```python
from build123d import *

# Parameters (mm, degrees)
F1_DEPTH = 2
F3_DEPTH = 26
F4_R     = 5


with BuildPart() as f1:
    # F0 (on Front) → F1 (new body)
    with BuildSketch(Plane.XZ):
        with BuildLine():
            Line((-15.958655, 29.411045), (-23, 0))
            Line((-23, 0), (23, 0))
            Line((23, 0), (15.958655, 29.411045))
            ThreePointArc((15.958655, 29.411045), (0, 42), (-15.958655, 29.411045))
        make_face()
        with BuildLine():
            Line((-9.25, 20.25), (-9.25, 26.75))
            ThreePointArc((-9.25, 26.75), (0, 36), (9.25, 26.75))
            Line((9.25, 26.75), (9.25, 20.25))
            ThreePointArc((9.25, 20.25), (0, 11), (-9.25, 20.25))
        make_face(mode=Mode.SUBTRACT)
    extrude(amount=F1_DEPTH)

    # F2 (on face) → F3 (join)
    with BuildSketch(Plane(origin=(0, 0, 0), x_dir=(-1, 0, 0), z_dir=(0, 1, 0))):
        Polygon((22.521177, 2), (-22.521177, 2), (-23, 0), (23, 0), align=None)
    extrude(amount=F3_DEPTH)

    # F4
    f4_edges = [f1.edges().sort_by_distance(p)[0] for p in [
        (0, -2, 0),
        (0, 0, 2),
    ]]
    fillet(f4_edges, radius=F4_R)


solid = f1.part
```
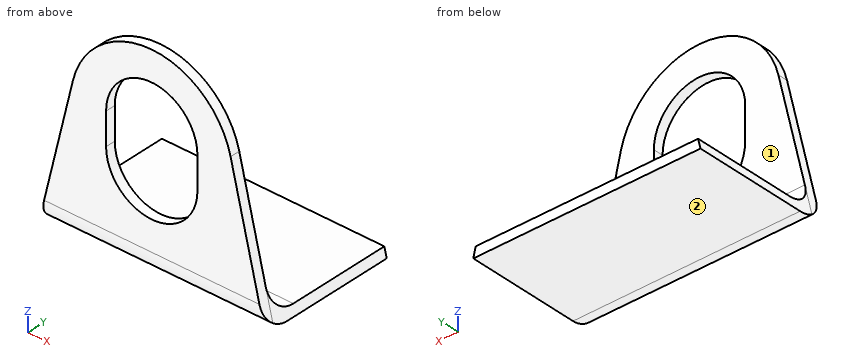
Source: CAD feature listing. Evaluate the final solid. Frame: model axes, mm. Face numbers are marked on the shaded views. A direction names the side the tool comes from. Give positions to 0.01 mm unless a question says otherwise; leave off trailing zeros. Write each loop counter-clockwise with the first axis right and the second up, starting at its lowest first coordinate (ties: lowest second). Pieces come first, ordered by that corner, then holes.
1. Section query D-D (z = 24.5). Return the cut outline in (x, y), then the cut area to 3 significant figures.
2. Material intervals for line 1 along Y through (x, z) = (9.5, 34); line 2 along Z through (x, y) = (3.5, 14); line 3 along Y through (x, z) = (12.5, 6), sorted ascending.
3. Section query B-B (z = 16). Return the cut outline in (x, y).
4. Section query A-A (x = 0). Return the cut outline in (y, z).
5. Section query C-C (y = 17.25). Return the cut outline in (x, z), then the cut area to 3 significant figures.
6. First-contact query: pin 1 (17.5 mm diameter, centred on x = -6, z = 17.5, fed in from +Y); pin 2 (1 mm diameter, centred on y = -1.5, z = 25, fed in from +X); pin 3 (6.5 mm diameter, centred on x = 2, y = 15, fed in from +Z). Flat tips, straight axial feed; report the tip coordinate or a pass-through.
7. Access query for the marked faces 1 and 2. Directions: +Z, -Z, +X, -X, +Y, -Y. A direction counts if a zero-diameter tool reaches every point of the face in a straight line with its end or side. Return the directions, or none.
Output values:
1. outline: (-17.13, -2) - (-9.25, -2) - (-9.25, 0) - (-17.13, 0) - close; (9.25, -2) - (17.13, -2) - (17.13, 0) - (9.25, 0) - close
1. area: 31.5 mm2
2. line 1: y = -2 to 0
2. line 2: z = 0 to 2
2. line 3: y = -2 to 0.1
3. outline: (-19.17, -2) - (-8.22, -2) - (-8.22, 0) - (-19.17, 0) - close; (8.22, -2) - (19.17, -2) - (19.17, 0) - (8.22, 0) - close
4. outline: (-2, 5) arc R5 ccw to (3, 0) - (26, 0) - (26, 2) - (5, 2) arc R5 cw to (0, 7) - (0, 11) - (-2, 11) - close; (-2, 36) - (0, 36) - (0, 42) - (-2, 42) - close
5. outline: (-23, 0) - (23, 0) - (22.52, 2) - (-22.52, 2) - close
5. area: 91.0 mm2
6. pin 1: stops at y = 0
6. pin 2: stops at x = 17.13
6. pin 3: stops at z = 2
7. face 1: +Z, +X, -X, +Y
7. face 2: -Z, +X, -X, +Y, -Y
